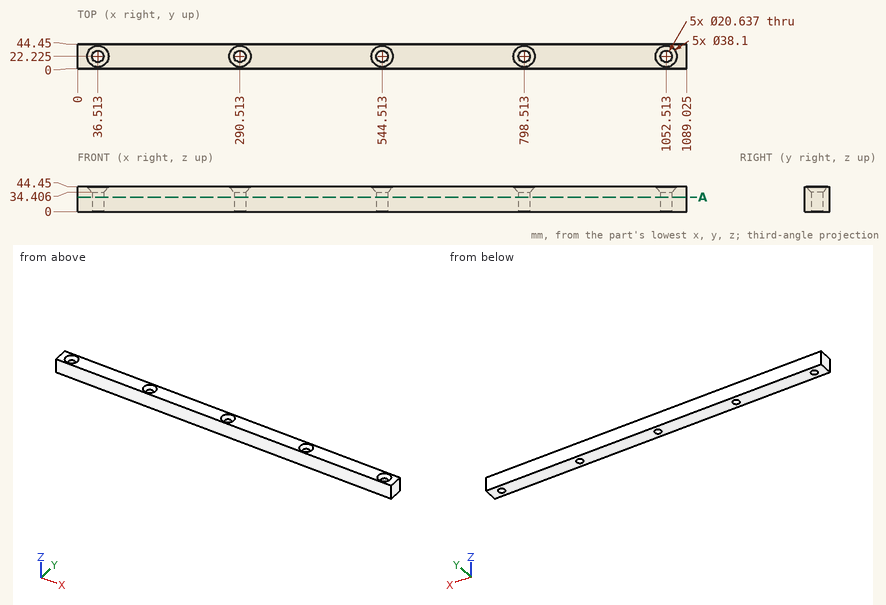
Here's the drawing with two shaded views (mm, measured from the low corner). I have some questions. Give positions to 0.01 mm unless a question says otherwise; leave off trailing zeros. Use one line per item in the form item = value. Start each with the question number.
(1) I'm going to push a flat-ended pin straight in: P1, Ø23.5, axis at x = 798.51, y = 22.22, coming from the +Z side. Where does the tip first touch, or does it pass through?
(2) Please list where these lines run through material, in increasing order: line 1 (X direction, y = 24, z = 13) (1 decimal); line 2 (X direction, y = 17.5, z = 37) (1 decimal); line 3 (Y direction, x = 538, z = 20).
(3) I want a section at A-A, the plane z = 26. State how many separate pieces and enclosed holes the cut face has, and give its area (3 significant figures).
Worked out:
q1.P1 = 36.06
q2.line_1 = 0 to 26.3, 46.7 to 280.3, 300.7 to 534.3, 554.7 to 788.3, 808.7 to 1042.3, 1062.7 to 1089
q2.line_2 = 0 to 24.9, 48.2 to 278.9, 302.2 to 532.9, 556.2 to 786.9, 810.2 to 1040.9, 1064.2 to 1089
q2.line_3 = 0 to 14.22, 30.23 to 44.45
q3.separate_pieces = 1
q3.enclosed_holes = 5
q3.area = 46,700 mm²
